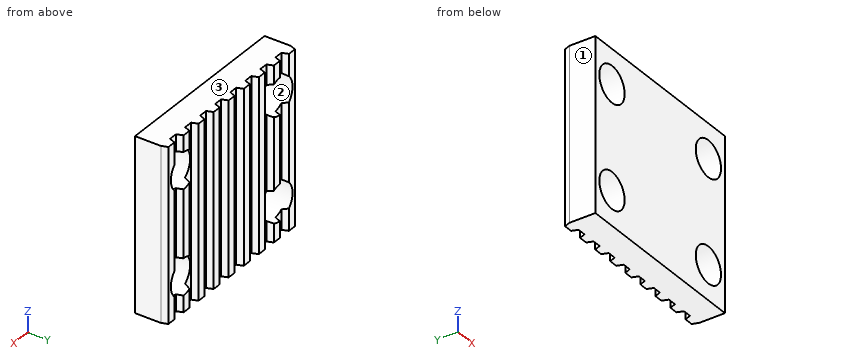
```python
from build123d import *

# Parameters (mm, degrees)
BOSS_EXTRUDE1_DEPTH = 10
SKETCH2_R           = 2.1
CUT_EXTRUDE1_DEPTH  = 4.7


with BuildPart() as part:
    # Sketch1 → Boss-Extrude1 (new body, symmetric)
    with BuildSketch(Plane.XY):
        Polygon((-10.754779164, 1.5), (-10.5, 2.2), (-9.5, 2.2), (-9.245220836, 1.5), (-8.254779164, 1.5), (-8, 2.2), (-7, 2.2), (-6.745220836, 1.5), (-5.754779164, 1.5), (-5.5, 2.2), (-4.5, 2.2), (-4.245220836, 1.5), (-3.254779164, 1.5), (-3, 2.2), (-2, 2.2), (-1.745220836, 1.5), (-0.754779164, 1.5), (-0.5, 2.2), (0.5, 2.2), (0.754779164, 1.5), (1.745220836, 1.5), (2, 2.2), (3, 2.2), (3.254779164, 1.5), (4.245220836, 1.5), (4.5, 2.2), (5.5, 2.2), (5.754779164, 1.5), (6.745220836, 1.5), (7, 2.2), (8, 2.2), (8.254779164, 1.5), (9.245220836, 1.5), (9.5, 2.2), (10.5, 2.2), (10.754779164, 1.5), (10.754779164, -1.5), (-10.754779164, -1.5), align=None)
    extrude(amount=BOSS_EXTRUDE1_DEPTH, both=True)

    # Sketch2 → Cut-Extrude1 (cut, through all)
    with BuildSketch(Plane.XZ.offset(1.5)):
        with Locations((-8, -6)):
            Circle(SKETCH2_R)
        with Locations((8, -6)):
            Circle(SKETCH2_R)
        with Locations((8, 6)):
            Circle(SKETCH2_R)
        with Locations((-8, 6)):
            Circle(SKETCH2_R)
    extrude(amount=-CUT_EXTRUDE1_DEPTH, mode=Mode.SUBTRACT)


solid = part.part
```
Check sheet for the modelled part. Datum: model origin and axes. Units: mm. Face numbers are marked on the shaded views. Round coordinates to 2 decimals unless told otherwise and drop trailing zeros. Loops run counter-clockwise (first coordinate to the right, second up) from the corner with the lowest first, then second, coordinate; pieces in that order, holes last. Notation, with made-up numbers: (-38.75, -25) -> (-16.75, -25) arc R8 cw to (-16.75, -21) -> close; hole circle Ø3 at (-39, 76). An arc over 180 degrees is marked (long way). Write item = value, one per line. Start each with the question number.
1) Gauge pin test, flat end, axial feed: pin 1 Ø4 at (x, z) = (-8, -6) entering from +Y. Record the tip position at first contact, or that the pin passes through.
2) Sectioned sample at A-A, the plane y = -1.2. Record the cut outline in (x, z).
3) Sectioned sample at B-B, the plane z = 6. State how many separate pieces and enclosed holes the cut face has, plus the area to 3 significant figures.
4) Thickness scan on probe 1 along Z at (x, y) = (-8, 0); probe 2 along X at (y, z) = (-0.1, 6); probe 3 along X at (y, z) = (-0.1, -5.5). Record the ranges inside material, lowest first.
5) Release check for a two-part mould opening along X. For the marked faces 1, 2 and 3 record: released by +X, released by -X, zero draft, split by the parting line, or undercut.
Results are:
q1.pin_1 = through
q2.outline = (-10.75, -10) -> (10.75, -10) -> (10.75, 10) -> (-10.75, 10) -> close; hole circle Ø4.2 at (-8, -6); hole circle Ø4.2 at (-8, 6); hole circle Ø4.2 at (8, -6); hole circle Ø4.2 at (8, 6)
q3.separate_pieces = 3
q3.enclosed_holes = 0
q3.area = 44.5 mm^2
q4.probe_1 = -10 to -8.1, -3.9 to 3.9, 8.1 to 10
q4.probe_2 = -10.75 to -10.1, -5.9 to 5.9, 10.1 to 10.75
q4.probe_3 = -10.75 to -10.04, -5.96 to 5.96, 10.04 to 10.75
q5.face_1 = released by -X
q5.face_2 = undercut
q5.face_3 = zero draft
